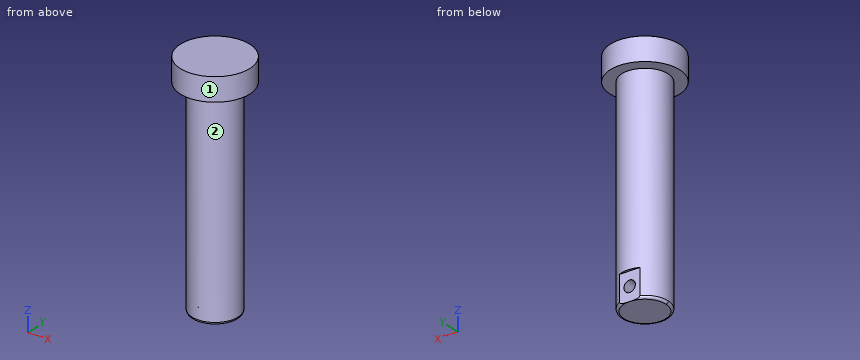
Autodesk Inventor part; units mm, degrees
ref_plane "YZ Plane" through (0, 0, 0) normal (1, 0, 0) x (0, 1, 0)
ref_plane "XZ Plane" through (0, 0, 0) normal (0, 1, 0) x (-1, 0, 0)
ref_plane "XY Plane" through (0, 0, 0) normal (0, 0, 1) x (1, 0, 0)
sketch "Sketch1" plane through (0, 0, 0) normal (0, 0, 1) x (1, 0, 0)
  circle A0 centre (0, 0) radius 7.5
extrude "Extrusion1" add sketch "Sketch1" along normal blind 5
sketch "Sketch2" plane through (0, 0, 0) normal (0, 0, -1) x (-1, 0, 0)
  circle A0 centre (0, 0) radius 5
extrude "Extrusion2" add sketch "Sketch2" along normal blind 45
fillet "Fillet1" radius 0.5 1 edges at (5, 0, -45)
sketch "Sketch3" plane through (0, 0, -45) normal (0, 0, -1) x (-1, 0, 0)
  point P0 (0, 0)
sketch "Sketch4" plane through (0, 0, -45) normal (0, 0, -1) x (-1, 0, 0)
  line L0 (0, 4.5) -> (5, 4.5)
  line L1 (5, 4.5) -> (5, 5.5)
  line L2 (5, 5.5) -> (-5, 5.5)
  line L3 (-5, 5.5) -> (-5, 4.5)
  line L4 (-5, 4.5) -> (0, 4.5)
  circle A0 centre (0, 0) radius 4.5
extrude "Extrusion3" cut sketch "Sketch4" against normal blind 6 contours L4 L3 L2 L1 L0
sketch "Sketch5" plane through (-2.1794, 4.5, -39) normal (0, 1, 0) x (1, 0, 0)
  point P0 (2.1794, -39)
  point P1 (2.1794, 6)
sketch "Sketch6" plane through (-2.1794, 4.5, -39) normal (0, 1, 0) x (1, 0, 0)
  point P0 (2.1794, -39)
sketch "Sketch7" plane through (-2.1794, 4.5, -39) normal (0, 1, 0) x (1, 0, 0)
  point P0 (2.1794, -39)
sketch "Sketch8" plane through (-2.1794, 4.5, -39) normal (0, 1, 0) x (1, 0, 0)
  point P0 (2.1794, -39)
  point P1 (2.1794, -3)
  point P2 (2.1794, -3)
  point P3 (2.1794, 3)
hole "Hole1" at (0, 4.5, -42) direction (0, -1, 0) diameter 2.459 depth 8.8 tip angle 118
properties part number "Trzemień"
Could you check a few things on this model? Use its own coordinates, in mm. Face numbers are marked on the shaded views. A direction names the side the tool comes from. Give positions to 0.01 mm unless a question says otherwise; leave off trailing zeros. Order: outer loops, then holes, each group sorted by start corner. A loop starts at its lowest first (then second) coordinate and runs counter-clockwise, first axis right, second up. Notation, with made-up numbers: (-36, 49) -> (-5, 49) arc R23 cw to (-5, 64) -> close; hole circle Ø8 at (-4.75, -13.75). An arc over 180 degrees is marked (long way). Answer in a Markdown table with one row per item. Add a question column.
Item 1: Please list where these lines run through material, in increasing order: probe 1 along Z at (x, y) = (0, -0.25); probe 2 along Z at (x, y) = (5.25, -3); probe 3 along X at (y, z) = (2.75, -42).
Item 2: Imagine slicing it at A-A (z = -26). List the corners of the cut face in (x, y) for me.
Item 3: Imagine slicing it at B-B (y = -6). List the corners of the cut face in (x, z) for me, and give its area (3 significant figures).
Item 4: For the marked faces 1 and 2, which set-ups out of +Z, -Z, +X, -X, +Y, -Y let a thin tool reach every point of the face, with its end or its side?
Item 5: I'm going to push flat-ended pins straight in: P1, Ø2, axis at y = 1.5, z = -4, coming from the -X side; P2, Ø1, axis at y = 5, z = -6, coming from the -X side; P3, Ø4, axis at x = -5, z = -30, coming from the -Y side. Where does each tip first touch, or does it pass through?
Item 6: Imagine slicing it at C-C (y = 6.25). List the corners of the cut face in (x, z) for me, and give its area (3 significant figures).
Result:
| question | item | result |
|---|---|---|
| 1 | probe 1 | -45 to -43.23, -40.77 to 5 |
| 1 | probe 2 | 0 to 5 |
| 1 | probe 3 | -4.18 to -1.23, 1.23 to 4.18 |
| 2 | outline | circle Ø10 at (0, 0) |
| 3 | outline | (-4.5, 0) -> (4.5, 0) -> (4.5, 5) -> (-4.5, 5) -> close |
| 3 | area | 45.0 mm2 |
| 4 | face 1 | +Z, -Z |
| 4 | face 2 | -Z |
| 5 | P1 | x = -4.97 |
| 5 | P2 | x = -2.18 |
| 5 | P3 | y = -4 |
| 6 | outline | (-4.15, 0) -> (4.15, 0) -> (4.15, 5) -> (-4.15, 5) -> close |
| 6 | area | 41.5 mm2 |
